Input: part model. Units: mm. Frame: model coordinates. A direction names the side the tool comes from. Give positions to 0.01 mm unless a question says otherwise; leave off trailing zeros. Write each loop counter-clockwise with the first axis right and the second up, starting at its lowest first coordinate (ties: lowest second). Pieces come first, ordered by that corner, then holes.
```python
from build123d import *

# Parameters (mm, degrees)
F1_DEPTH      = 10
F3_DEPTH      = 10
F3_DEPTH_BACK = 8
F4_R          = 5
F5_R          = 2.99999


# Not quite as in the source:
# - a fillet or chamfer is up to 0.001 mm smaller than in the source, because OpenCascade refuses the exact size


with BuildPart() as f1:
    # F0 (on Front) → F1 (new body)
    with BuildSketch(Plane.XZ):
        Polygon((38, 0), (0, 0), (0, -38), (6, -38), (6, -6), (38, -6), align=None)
    extrude(amount=F1_DEPTH)

    # F2 (on Front) → F3 (cut, two sides)
    with BuildSketch(Plane.XZ) as f3_sk:
        Polygon((36, -2), (2, -2), (2, -36), (4, -36), (4, -4), (36, -4), align=None)
    extrude(amount=-F3_DEPTH, mode=Mode.SUBTRACT)
    extrude(f3_sk.sketch, amount=F3_DEPTH_BACK, mode=Mode.SUBTRACT)

    # F4
    f4_edges = [f1.edges().sort_by_distance(p)[0] for p in [
        (0, -5, 0),
        (4, -4, -4),
        (2, -4, -2),
        (6, -5, -6),
    ]]
    fillet(f4_edges, radius=F4_R)

    # F5 (radius 3 in the source; OpenCascade refuses exactly that, so slightly less here)
    f5_edges = [f1.edges().sort_by_distance(p)[0] for p in [
        (3, -10, -38),
        (6, -10, -24.5),
        (21.5, -10, 0),
        (38, -10, -3),
    ]]
    fillet(f5_edges, radius=F5_R)


solid = f1.part
```
Item 1: Set-up query: faces 4 (the flat face through (24, -3, -6)), 5 (the flat face through (38, -3, -3)), 6 (the flat face through (2, -4, -21)). Return all of +Z, -Z, +X, -X, +Y, -Y with unobstructed straight access to the full face (end or side cutting, diameter ignored); none if empty.
Item 2: Ray query, line 1 (Z direction, x = 29.5, y = -6.25); line 2 (X direction, y = -1.5, z = -14.5); line 3 (Z direction, x = 3, y = -7.5). Return the intervals inside material, ascending.
Item 3: Mould query, pull axis X, two halves, no side actions, for faces 1 (the flat face through (4, -4, -23)), 2 (the cylindrical face through (0.86, -9.1, -21.73)), 3 (the cylindrical face through (3.042, -8.748, -37.438)). Classes: +X half, -X half, draft (parallel to the pull), parting line (faces both ways), or undercut.
Item 4: Pin query (flat end, axial travel): pin 1 (1.6 mm diameter, centred on y = -5, z = -3, fed in from -X); pin 2 (2 mm diameter, centred on x = 7.5, z = -13, fed in from +Y); pin 3 (1 mm diameter, centred on x = 3, y = -5, fed in from +Z); pin 4 (1.5 mm diameter, centred on x = 33.5, y = -9, fed in from -Z). Return the tip coordinate at first contact, or that it passes through.
Item 5: Section A-A (y = -5.75). Return loops of the section in (x, z), and give its area (3 significant figures).
Solved:
1. face 4: -Z, +X, +Y, -Y
1. face 5: +Z, -Z, +X, +Y, -Y
1. face 6: +Y
2. line 1: z = -6 to -4, -2 to 0
2. line 2: x = 0 to 2, 4 to 6
2. line 3: z = -37.96 to -36, -4 to -0.46
3. face 1: undercut
3. face 2: -X half
3. face 3: draft
4. pin 1: stops at x = 0.15
4. pin 2: passes through
4. pin 3: stops at z = -0.23
4. pin 4: stops at z = -5.73
5. outline: (0, -38) - (6, -38) - (6, -11) arc R5 cw to (11, -6) - (38, -6) - (38, 0) - (5, 0) arc R5 ccw to (0, -5) - close; hole (2, -36) - (4, -36) - (4, -9) arc R5 cw to (9, -4) - (36, -4) - (36, -2) - (7, -2) arc R5 ccw to (2, -7) - close
5. area: 288 mm2
